from build123d import *

# Parameters (mm, degrees)
SKETCH1_W                = 55.88
SKETCH1_H                = 55.88
BOSS_EXTRUDE1_DEPTH      = 50.8
SKETCH2_W                = 43.18
SKETCH2_H                = 38.1
CUT_EXTRUDE1_DEPTH       = 56.88
SKETCH3_W                = 43.18
SKETCH3_H                = 38.1
CUT_EXTRUDE2_DEPTH       = 56.88
SKETCH4_R                = 1.75
SKETCH4_W                = 25.4
SKETCH4_H                = 25.4
CUT_EXTRUDE3_DEPTH       = 44.45
BOSS_EXTRUDE2_DEPTH      = 3.175
BOSS_EXTRUDE2_DEPTH_BACK = 3.175
SKETCH10_W               = 9.525
SKETCH10_H               = 3.175
BOSS_EXTRUDE5_DEPTH      = 55.88
SKETCH12_W               = 62.23
SKETCH12_H               = 3.175
BOSS_EXTRUDE6_DEPTH      = 3.175
BOSS_EXTRUDE6_DEPTH_BACK = 6.35
SKETCH13_W               = 62.23
SKETCH13_H               = 3.175
BOSS_EXTRUDE7_DEPTH      = 3.175
BOSS_EXTRUDE7_DEPTH_BACK = 6.35
SKETCH11_R               = 1.75
SKETCH11_R_2             = 1.778
CUT_EXTRUDE4_DEPTH       = 48.625
SKETCH15_R               = 2.54
SKETCH15_R_2             = 1.75
SKETCH15_R_3             = 1.778
BOSS_EXTRUDE8_DEPTH      = 7.239
SKETCH16_R               = 1.651
BOSS_EXTRUDE9_DEPTH      = 3.175


with BuildPart() as part:
    # Sketch1 → Boss-Extrude1 (new body)
    with BuildSketch(Plane(origin=(0, 0, 0), x_dir=(1, 0, 0), z_dir=(0, 1, 0))):
        with Locations((27.94, 27.94)):
            Rectangle(SKETCH1_W, SKETCH1_H)
    extrude(amount=BOSS_EXTRUDE1_DEPTH)

    # Sketch2 → Cut-Extrude1 (cut, through all)
    with BuildSketch(Plane.XY):
        with Locations((27.94, 25.4)):
            Rectangle(SKETCH2_W, SKETCH2_H)
    extrude(amount=-CUT_EXTRUDE1_DEPTH, mode=Mode.SUBTRACT)

    # Sketch3 → Cut-Extrude2 (cut, through all)
    with BuildSketch(Plane(origin=(55.88, 0, 0), x_dir=(0, 0, -1), z_dir=(1, 0, 0))):
        with Locations((27.94, 25.4)):
            Rectangle(SKETCH3_W, SKETCH3_H)
    extrude(amount=-CUT_EXTRUDE2_DEPTH, mode=Mode.SUBTRACT)

    # Sketch4 → Cut-Extrude3 (cut)
    with BuildSketch(Plane(origin=(0, 50.8, 0), x_dir=(1, 0, 0), z_dir=(0, 1, 0))):
        with Locations((43.44, 43.44)):
            Circle(SKETCH4_R)
        with Locations((43.44, 12.44)):
            Circle(SKETCH4_R)
        with Locations((12.44, 12.44)):
            Circle(SKETCH4_R)
        with Locations((12.44, 43.44)):
            Circle(SKETCH4_R)
        with Locations((27.94, 27.94)):
            Rectangle(SKETCH4_W, SKETCH4_H)
    extrude(amount=-CUT_EXTRUDE3_DEPTH, mode=Mode.SUBTRACT)

    # Sketch5 → Cut-Revolve1 (revolve, cut)
    with BuildSketch(Plane(origin=(12.44, 0, 0), x_dir=(0, 0, -1), z_dir=(1, 0, 0))):
        Polygon((43.44, 50.8), (40.138, 50.8), (43.44, 47.498), align=None)
    revolve(axis=Axis((12.44, 47.498, -43.44), (0, 1, 0)), mode=Mode.SUBTRACT)

    # Sketch6 → Cut-Revolve2 (revolve, cut)
    with BuildSketch(Plane(origin=(12.44, 0, 0), x_dir=(0, 0, -1), z_dir=(1, 0, 0))):
        Polygon((12.44, 50.8), (9.138, 50.8), (12.44, 47.498), align=None)
    revolve(axis=Axis((12.44, 47.498, -12.44), (0, 1, 0)), mode=Mode.SUBTRACT)

    # Sketch7 → Cut-Revolve3 (revolve, cut)
    with BuildSketch(Plane(origin=(43.44, 0, 0), x_dir=(0, 0, -1), z_dir=(1, 0, 0))):
        Polygon((43.44, 50.8), (40.138, 50.8), (43.44, 47.498), align=None)
    revolve(axis=Axis((43.44, 47.498, -43.44), (0, 1, 0)), mode=Mode.SUBTRACT)

    # Sketch8 → Cut-Revolve4 (revolve, cut)
    with BuildSketch(Plane(origin=(43.44, 0, 0), x_dir=(0, 0, -1), z_dir=(1, 0, 0))):
        Polygon((12.44, 50.8), (9.138, 50.8), (12.44, 47.498), align=None)
    revolve(axis=Axis((43.44, 47.498, -12.44), (0, 1, 0)), mode=Mode.SUBTRACT)

    # Sketch9 → Boss-Extrude2 (add, two sides)
    with BuildSketch(Plane.XZ.offset(-44.45)) as boss_extrude2_sk:
        with BuildLine():
            Line((0, -40.64), (0, -15.24))
            ThreePointArc((0, -15.24), (-1.005581006, -19.499709497), (-3.81, -22.86))
            ThreePointArc((-3.81, -22.86), (-6.35, -27.94), (-3.81, -33.02))
            ThreePointArc((-3.81, -33.02), (-1.005581006, -36.380290503), (0, -40.64))
        make_face()
        with BuildLine():
            Line((55.88, -40.64), (55.88, -15.24))
            ThreePointArc((55.88, -15.24), (56.885581006, -19.499709497), (59.69, -22.86))
            ThreePointArc((59.69, -22.86), (62.23, -27.94), (59.69, -33.02))
            ThreePointArc((59.69, -33.02), (56.885581006, -36.380290503), (55.88, -40.64))
        make_face()
        with BuildLine():
            Line((15.24, 0), (40.64, 0))
            ThreePointArc((40.64, 0), (36.380290503, 1.005581006), (33.02, 3.81))
            ThreePointArc((33.02, 3.81), (27.94, 6.35), (22.86, 3.81))
            ThreePointArc((22.86, 3.81), (19.499709497, 1.005581006), (15.24, 0))
        make_face()
        with BuildLine():
            Line((15.24, -55.88), (40.64, -55.88))
            ThreePointArc((40.64, -55.88), (36.380290503, -56.885581006), (33.02, -59.69))
            ThreePointArc((33.02, -59.69), (27.94, -62.23), (22.86, -59.69))
            ThreePointArc((22.86, -59.69), (19.499709497, -56.885581006), (15.24, -55.88))
        make_face()
    extrude(amount=BOSS_EXTRUDE2_DEPTH)
    extrude(boss_extrude2_sk.sketch, amount=-BOSS_EXTRUDE2_DEPTH_BACK)

    # Sketch10 → Boss-Extrude5 (add)
    with BuildSketch(Plane.XY):
        with Locations((54.2925, 42.8625)):
            Rectangle(SKETCH10_W, SKETCH10_H)
        with Locations((1.5875, 42.8625)):
            Rectangle(SKETCH10_W, SKETCH10_H)
    extrude(amount=-BOSS_EXTRUDE5_DEPTH)

    # Sketch12 → Boss-Extrude6 (add, two sides)
    with BuildSketch(Plane(origin=(0, 0, -55.88), x_dir=(-1, 0, 0), z_dir=(0, 0, -1))) as boss_extrude6_sk:
        with Locations((-27.94, 42.8625)):
            Rectangle(SKETCH12_W, SKETCH12_H)
    extrude(amount=BOSS_EXTRUDE6_DEPTH)
    extrude(boss_extrude6_sk.sketch, amount=-BOSS_EXTRUDE6_DEPTH_BACK)

    # Sketch13 → Boss-Extrude7 (add, two sides)
    with BuildSketch(Plane.XY) as boss_extrude7_sk:
        with Locations((27.94, 42.8625)):
            Rectangle(SKETCH13_W, SKETCH13_H)
    extrude(amount=BOSS_EXTRUDE7_DEPTH)
    extrude(boss_extrude7_sk.sketch, amount=-BOSS_EXTRUDE7_DEPTH_BACK)

    # Sketch11 → Cut-Extrude4 (cut, through all)
    with BuildSketch(Plane(origin=(0, 47.625, 0), x_dir=(1, 0, 0), z_dir=(0, 1, 0))):
        with Locations((-3.81, 27.94)):
            Circle(SKETCH11_R)
        with Locations((59.69, 27.94)):
            Circle(SKETCH11_R)
        with Locations((27.94, -3.81)):
            Circle(SKETCH11_R_2)
        with Locations((27.94, 59.69)):
            Circle(SKETCH11_R_2)
    extrude(amount=-CUT_EXTRUDE4_DEPTH, mode=Mode.SUBTRACT)

    # Sketch14 → Revolve1 (revolve)
    with BuildSketch(Plane(origin=(0, 0, -27.94), x_dir=(-1, 0, 0), z_dir=(0, 0, -1))):
        with BuildLine():
            Line((-8.89, 0), (-24.765, -2.888501777))
            ThreePointArc((-24.765, -2.888501777), (-26.346050014, -3.103230235), (-27.94, -3.175))
            Line((-27.94, -3.175), (-27.94, 0))
            Line((-27.94, 0), (-8.89, 0))
        make_face()
    revolve(axis=Axis((27.94, -3.175, -27.94), (0, 1, 0)))

    # Sketch15 → Boss-Extrude8 (add)
    with BuildSketch(Plane.XZ.offset(-41.275)):
        with Locations((-3.81, -27.94)):
            Circle(SKETCH15_R)
        with Locations((-3.81, -27.94)):
            Circle(SKETCH15_R_2, mode=Mode.SUBTRACT)
        with Locations((27.94, -59.69)):
            Circle(SKETCH15_R)
        with Locations((27.94, -59.69)):
            Circle(SKETCH15_R_3, mode=Mode.SUBTRACT)
    extrude(amount=BOSS_EXTRUDE8_DEPTH)

    # Sketch16 → Boss-Extrude9 (add)
    with BuildSketch(Plane.XZ.offset(-34.036)):
        with BuildLine():
            Line((34.29, -62.23), (21.59, -62.23))
            ThreePointArc((21.59, -62.23), (19.05, -59.69), (21.59, -57.15))
            Line((21.59, -57.15), (34.29, -57.15))
            ThreePointArc((34.29, -57.15), (36.83, -59.69), (34.29, -62.23))
        make_face()
        with Locations((34.29, -59.69)):
            Circle(SKETCH16_R, mode=Mode.SUBTRACT)
        with Locations((21.59, -59.69)):
            Circle(SKETCH16_R, mode=Mode.SUBTRACT)
        with BuildLine():
            Line((-6.35, -34.29), (-6.35, -21.59))
            ThreePointArc((-6.35, -21.59), (-3.81, -19.05), (-1.27, -21.59))
            Line((-1.27, -21.59), (-1.27, -34.29))
            ThreePointArc((-1.27, -34.29), (-3.81, -36.83), (-6.35, -34.29))
        make_face()
        with Locations((-3.81, -34.29)):
            Circle(SKETCH16_R, mode=Mode.SUBTRACT)
        with Locations((-3.81, -21.59)):
            Circle(SKETCH16_R, mode=Mode.SUBTRACT)
    extrude(amount=BOSS_EXTRUDE9_DEPTH)


solid = part.part
Verification items for the finished model (mm, model axes). A direction names the side the tool comes from. Round coordinates to 2 decimals unless told otherwise and drop trailing zeros. Loops run counter-clockwise (first coordinate to the right, second up) from the corner with the lowest first, then second, coordinate; pieces in that order, holes last. Notation, with made-up numbers: M -2.5,7 L 47.5,7 A28 ccw 47.5,31 Z; hole C 18.25,-12 d11. An arc over 180 degrees is marked long. Write each question's results on one line, items separated by ' | '.
1) Section check A-A on y = 43. Record the boundary of the cut face in (x, z) (3 decimals), then the cut area to 3 significant figures.
Checks:
outline: M -3.81,-33.02 A9.525 cw -3.175,-33.54 L -3.175,-59.055 L 22.34,-59.055 A9.525 cw 22.86,-59.69 A6.35 ccw 33.02,-59.69 A9.525 cw 33.54,-59.055 L 59.055,-59.055 L 59.055,-33.54 A9.525 cw 59.69,-33.02 A6.35 ccw 59.69,-22.86 A9.525 cw 59.055,-22.34 L 59.055,3.175 L 33.54,3.175 A9.525 cw 33.02,3.81 A6.35 ccw 22.86,3.81 A9.525 cw 22.34,3.175 L -3.175,3.175 L -3.175,-22.34 A9.525 cw -3.81,-22.86 A6.35 ccw Z; hole C -3.81,-27.94 d3.5; hole M 6.35,-49.53 L 49.53,-49.53 L 49.53,-6.35 L 6.35,-6.35 Z; hole C 27.94,-59.69 d3.556; hole C 27.94,3.81 d3.556; hole C 59.69,-27.94 d3.5 | area: 2,070 mm2
2) Section check D-D on x = 1. Record the boundary of the cut face in (y, z) (3 decimals).
Checks:
outline: M 0,-55.88 L 41.275,-55.88 L 41.275,-59.055 L 44.45,-59.055 L 44.45,-55.88 L 50.8,-55.88 L 50.8,0 L 44.45,0 L 44.45,3.175 L 41.275,3.175 L 41.275,0 L 0,0 Z; hole M 6.35,-49.53 L 41.275,-49.53 L 41.275,-6.35 L 6.35,-6.35 Z
3) Mould release check, pull along Z, two halves, no side actions. Record for faces 1 (the flat face through (-3.175, 43, -9)), 2 (the flat face through (28, 32, -62.23)), 3 (the flat face through (28, 48, -40.64)), 4 (the flat face through (14, 44.45, -28)): released by +Z, released by -Z, zero draft, split by the parting line, or undercut.
Checks:
face 1: zero draft | face 2: released by -Z | face 3: undercut | face 4: undercut
4) Scan lines: L1, parallel to X at y = 45.8, z = -43.44; L2, parallel to Z at x = 27.94, y = 44; L3, parallel to Z at x = -3.81, y = 32.8. Record each from-to range of solid material in increasing order. Write a range as from..to.
Checks:
L1: x = 0..10.69, 14.19..41.69, 45.19..55.88 | L2: z = -62.23..-61.47, -57.91..-49.53, -6.35..2.03, 5.59..6.35 | L3: z = -36.83..-35.94, -32.64..-23.24, -19.94..-19.05
5) Access from +Z, -Z, +X, -X, +Y, -Y to the whole of each face (thin tool, end or side, straight path). Record for faces 5 (the cylindrical face through (-5.027, 32.471, -20.474)), 6 (the cylindrical face through (45.057, 46.883, -11.77)), 7 (the flat face through (53, 24, -6.35)).
Checks:
face 5: -Y | face 6: +Y | face 7: +X, -X
6) Section check C-C on z = -3. Record the boundary of the cut face in (x, y) (3 decimals), then the cut area to 3 significant figures.
Checks:
outline: M -3.175,41.275 L 0,41.275 L 0,0 L 55.88,0 L 55.88,41.275 L 59.055,41.275 L 59.055,44.45 L 55.88,44.45 L 55.88,50.8 L 0,50.8 L 0,44.45 L -3.175,44.45 Z; hole M 6.35,6.35 L 49.53,6.35 L 49.53,41.275 L 6.35,41.275 Z | area: 1,350 mm2
7) Gauge pin test, flat ends, axial feed: P1, Ø1.6, axis at x = 29.5, y = 32, coming from the +Z side; P2, Ø7, axis at y = 48.5, z = -31.5, coming from the -X side; P3, Ø4, axis at x = -3.81, z = -34.29, coming from the -Y side; P4, Ø5, axis at x = 26, y = 46.5, coming from the +Z side. Record the tip position at first contact, or that the pin passes through.
Checks:
P1: stops at z = -57.15 | P2: stops at x = -6.35 | P3: stops at y = 30.86 | P4: stops at z = 6.35
8) Section check B-B on y = 20. Record the boundary of the cut face in (x, z).
Checks:
outline: M 0,-55.88 L 6.35,-55.88 L 6.35,-49.53 L 0,-49.53 Z; M 0,-6.35 L 6.35,-6.35 L 6.35,0 L 0,0 Z; M 49.53,-55.88 L 55.88,-55.88 L 55.88,-49.53 L 49.53,-49.53 Z; M 49.53,-6.35 L 55.88,-6.35 L 55.88,0 L 49.53,0 Z
